```python
from build123d import *

# Parameters (mm, degrees)
CHAMFER1_R      = 0.5
HOLE_DEPTH      = 49.520614205
HOLE_DEPTH_BACK = 49.520614205
SKETCH2_R       = 1.69


with BuildPart() as part:
    # Sketch1 → BaseBody (revolve)
    with BuildSketch(Plane.XY, mode=Mode.PRIVATE) as basebody_sk:
        with BuildLine():
            Line((47.5, 0), (0, 0))
            Line((0, 0), (0, 5.75))
            ThreePointArc((0, 5.75), (1.25, 7), (2.5, 5.75))
            Line((2.5, 5.75), (2.5, 5))
            Line((2.5, 5), (46, 5))
            Line((46, 5), (47.5, 4.133974596))
            Line((47.5, 4.133974596), (47.5, 0))
        make_face()
    revolve(basebody_sk.sketch.rotate(Axis((-19.830028721, 0, 0), (1, 0, 0)), 180), axis=Axis((-19.830028721, 0, 0), (1, 0, 0)))

    # Chamfer1
    chamfer1_edges = [part.edges().sort_by_distance(p)[0] for p in [
        (2.5, 5, 0),
    ]]
    fillet(chamfer1_edges, radius=CHAMFER1_R)

    # Sketch2 → Hole (cut, two sides: drawn at the far end of the back side and taken through both)
    with BuildSketch(Plane(origin=(0, 0, 0), x_dir=(1, 0, 0), z_dir=(0, 1, 0)).offset(-HOLE_DEPTH_BACK)):
        with Locations(Location((43.5, 0, 0), (0, 0, 270))):
            Circle(SKETCH2_R)
    extrude(amount=HOLE_DEPTH + HOLE_DEPTH_BACK, mode=Mode.SUBTRACT)


solid = part.part
```
Verification items for the finished model (mm, model axes). Round coordinates to 2 decimals unless told otherwise and drop trailing zeros. Order: outer loops, then holes, each group sorted by start corner. A loop starts at its lowest first (then second) coordinate and runs counter-clockwise, first axis right, second up.
1) Draft check along Z on faces 1 (the cylindrical face through (24.8, 1.08, 4.88)), 2 (the cylindrical face through (45.176, -0.069, -0.22)), 3 (the flat face through (47.5, 0, 0)). Enter one of: +Z half, -Z half, draft (parallel to the pull), parting line (faces both ways), or undercut.
Geometry says:
face 1: parting line
face 2: undercut
face 3: draft
2) Cross-section at A-A, the plane z = 0. Record the cut outline in (x, y).
Geometry says:
outline: (0, -5.75) arc R1.25 ccw to (2.5, -5.75) - (2.5, -5.5) arc R0.5 cw to (3, -5) - (41.81, -5) - (41.81, 5) - (3, 5) arc R0.5 cw to (2.5, 5.5) - (2.5, 5.75) arc R1.25 ccw to (0, 5.75) - close; (45.19, -5) - (46, -5) - (47.5, -4.13) - (47.5, 4.13) - (46, 5) - (45.19, 5) - close
3) Cross-section at B-B, the plane y = 0. Record the cut outline in (x, z), plus the area to 3 significant figures.
Geometry says:
outline: (0, -5.75) arc R1.25 ccw to (2.5, -5.75) - (2.5, -5.5) arc R0.5 cw to (3, -5) - (46, -5) - (47.5, -4.13) - (47.5, 4.13) - (46, 5) - (3, 5) arc R0.5 cw to (2.5, 5.5) - (2.5, 5.75) arc R1.25 ccw to (0, 5.75) - close; hole circle Ø3.38 at (43.5, 0)
area: 473 mm2
4) Cross-section at C-C, the plane x = 37.5. Record the cut outline in (y, z).
Geometry says:
outline: circle Ø10 at (0, 0)
5) Depth check by flat-ended pin: pin 1 (1.5 mm diameter, centred on y = -4.5, z = -2, fed in from +X); pin 2 (8 mm diameter, centred on x = 8, z = 4, fed in from -Y); pin 3 (2 mm diameter, centred on x = 39.5, z = -2.5, fed in from +Y). Enter the tip coordinate at first touch or a pass-through.
Geometry says:
pin 1: stops at x = 47.43
pin 2: stops at y = -5
pin 3: stops at y = 4.77
6) Cross-section at D-D, the plane x = 43.5. Record the cut outline in (y, z).
Geometry says:
outline: (-4.71, -1.69) arc R5 ccw to (4.71, -1.69) - close; (-4.71, 1.69) - (4.71, 1.69) arc R5 ccw to start
7) Material ranges on line 1 (X direction, y = 1.75, z = 0); line 2 (Z direction, x = 43.5, y = 1); line 3 (X direction, y = -0.25, z = 0.75), recorded low to high.
Geometry says:
line 1: x = 0 to 41.81, 45.19 to 47.5
line 2: z = -4.9 to -1.69, 1.69 to 4.9
line 3: x = 0 to 41.99, 45.01 to 47.5
